Answer from the drawing. Dimensions are ordinates in mm from the lowest x, y and z of the part. Round coordinates to 2 decimals unless told otherwise and drop trailing zeros. Loops run counter-clockwise (first coordinate to the right, second up) from the corner with the lowest first, then second, coordinate; pieces in that order, holes last. Notation, with made-up numbers: (81, 79.25) - (124, 79.25) arc R25 ccw to (124, 110.25) - close; hole circle Ø1 at (-14, 28.5). An arc over 180 degrees is marked (long way). Answer as CSV lines item,"result".
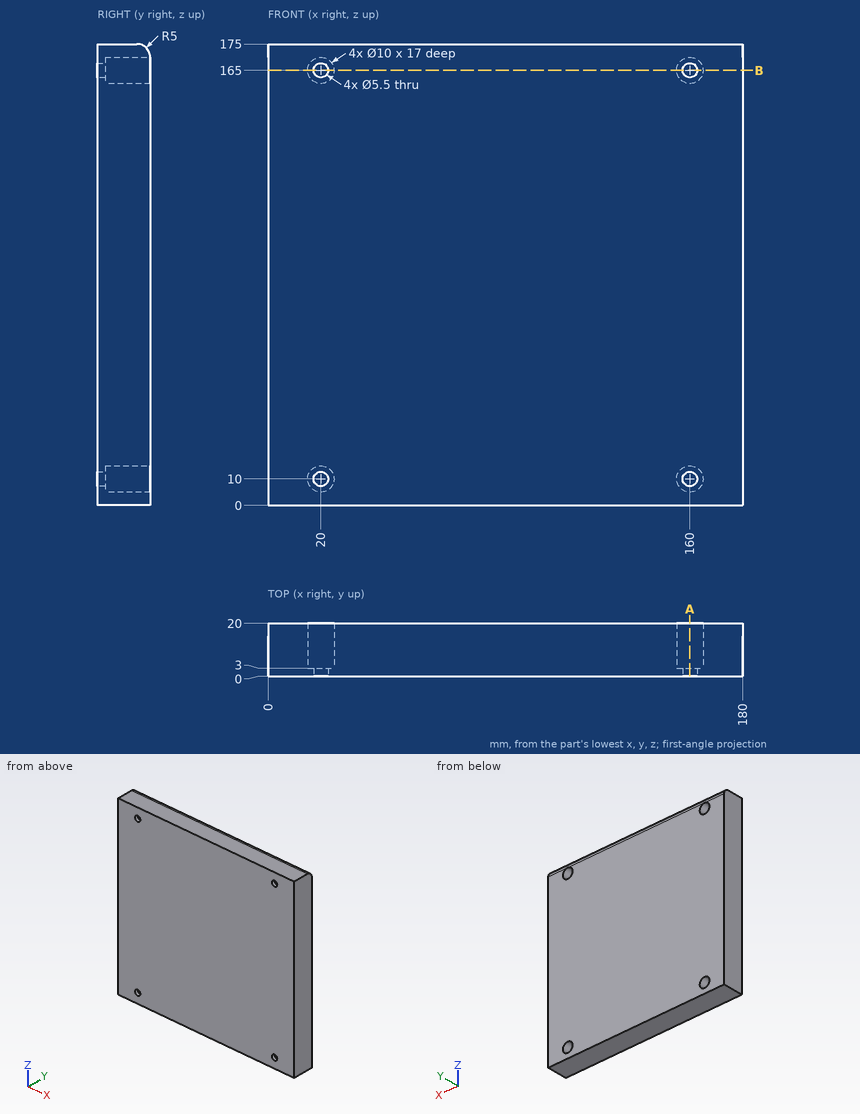
1) A cutting plane is placed at B-B, the plane z = 165. Determine the outline of the cut face in (x, y), plus the area to 3 significant figures.
Entries:
outline,"(0, 0) - (17.25, 0) - (17.25, 3) - (15, 3) - (15, 20) - (0, 20) - close; (22.75, 0) - (157.25, 0) - (157.25, 3) - (155, 3) - (155, 20) - (25, 20) - (25, 3) - (22.75, 3) - close; (162.75, 0) - (180, 0) - (180, 20) - (165, 20) - (165, 3) - (162.75, 3) - close"
area,"3,230 mm^2"
2) Find the intervals of material crossed by line 1 (Z direction, x = 19.5, y = 1.25); line 2 (X direction, y = 13, z = 165); line 3 (Z direction, x = 20, y = 12.5), in increasing order.
Entries:
line 1,"z = 0 to 7.3, 12.7 to 162.3, 167.7 to 175"
line 2,"x = 0 to 15, 25 to 155, 165 to 180"
line 3,"z = 0 to 5, 15 to 160, 170 to 175"
3) Each of these flat-tipped pins is pushed along its axis until it touches: P1, Ø12, axis at x = 115, y = 16, coming from the -Z side; P2, Ø5, axis at x = 22, z = 166, coming from the +Y side; P3, Ø3, axis at x = 20.5, y = 17, coming from the +Z side (3 decimals); P4, Ø1.5, axis at x = 61, y = 18, coming from the +Z side (3 decimals). Where does it stop, or does it pass through?
Entries:
P1,"stops at z = 0"
P2,"stops at y = 3"
P3,"stops at z = 174.975"
P4,"stops at z = 174.465"
4) A cutting plane is placed at A-A, the plane x = 160. Count the separate pieces of the cut face and the enclosed holes in it, plus the area to 3 significant figures.
Entries:
separate pieces,"3"
enclosed holes,"0"
area,"3,120 mm^2"
